```python
from build123d import *

# Parameters (mm, degrees)
F1_DEPTH = 2.25
F2_DEPTH = 2.55


with BuildPart() as f1:
    # F0 (on Top) → F1 (new body)
    with BuildSketch(Plane.XY):
        with BuildLine():
            ThreePointArc((-4.875, -1.5), (0, -0.2318236393), (4.875, -1.5))
            Line((4.875, -1.5), (4.875, 1.5))
            Line((4.875, 1.5), (-4.875, 1.5))
            Line((-4.875, 1.5), (-4.875, -1.5))
        make_face()
        with BuildLine():
            Line((1.0935325176, -1.5), (4.875, -1.5))
            ThreePointArc((4.875, -1.5), (0, -0.2318236393), (-4.875, -1.5))
            Line((-4.875, -1.5), (-1.0935325176, -1.5))
            ThreePointArc((-1.0935325176, -1.5), (0, -1.4318236393), (1.0935325176, -1.5))
        make_face()
    extrude(amount=F1_DEPTH)

    # F0 (on Top) → F2 (join)
    with BuildSketch(Plane.XY):
        with BuildLine():
            ThreePointArc((10.0040881804, -10.2359118196), (8.6270420829, -5.1707439823), (4.875, -1.5))
            Line((4.875, -1.5), (1.0935325176, -1.5))
            ThreePointArc((1.0935325176, -1.5), (6.6007395571, -4.4099178283), (8.8040881804, -10.2359118196))
            ThreePointArc((8.8040881804, -10.2359118196), (-5.8259939913, -16.8366513767), (-1.0935325176, -1.5))
            Line((-1.0935325176, -1.5), (-4.875, -1.5))
            ThreePointArc((-4.875, -1.5), (-5.0651678374, -18.8629539025), (10.0040881804, -10.2359118196))
        make_face()
    extrude(amount=F2_DEPTH)


solid = f1.part
```
The listing builds one solid part. Answer for the finished solid, in the listing's coordinates (mm). A direction names the side the tool comes from. Give positions to 0.01 mm unless a question says otherwise; leave off trailing zeros. Order: outer loops, then holes, each group sorted by start corner. A loop starts at its lowest first (then second) coordinate and runs counter-clockwise, first axis right, second up. Notation, with made-up numbers: (11, -14.5) -> (24, -14.5) arc R13 cw to (24, -6.5) -> close; hole circle Ø6 at (-27, -6). An arc over 180 degrees is marked (long way). Answer as a JSON object with one key per item and string values. Group by question number.
Item 1: The part is cut by section A-A on x = 0. Write down the section's boundary in (y, z).
Item 2: The part is cut by section C-C on z = 1.8. Write down the section's boundary in (x, y) (3 decimals), and give its area (3 significant figures).
Item 3: The part is cut by section B-B on y = -5.5. Write down the section's boundary in (x, z), and give its area (3 significant figures).
Item 4: Flat-ended cylindrical pins translate along their axes: pin 1 (1 mm diameter, centred on y = -4.5, z = 2, fed in from +X); pin 2 (2.5 mm diameter, centred on x = 1, y = 0.5, fed in from +Z); pin 3 (1.5 mm diameter, centred on y = -15, z = 1, fed in from +X); pin 4 (8 mm diameter, centred on x = 2, y = -8, fed in from -Z). Find the tip coordinate at first contact, or state that the pin passes through.
Item 5: Consider L1, parallel to Y at x = 0, z = 1.6; L2, parallel to X at y = -18.25, z = 0.2; L3, parallel to Y at x = 0.75, z = 2.2. Determine where each line is inside the solid, lowest interval first. Write a range as from..to.
Item 6: A tool of negligible diameter and unlimited length cuts with its end or side. For faces 1 (the flat face through (0, 1.5, 1)), 2 (the flat face through (0, 0, 2.25)), 3 (the flat face through (-0.8, -19.2, 2.55)), 4 (the flat face through (4.875, 0, 1)), 5 (the flat face through (-4.875, 0, 1)), from which of +Z, -Z, +X, -X, +Y, -Y can it reach the whole face along a straight path? Write none if from no direction.
Result set:
{
 "1": {"outline": "(-20.24, 0) -> (-19.04, 0) -> (-19.04, 2.55) -> (-20.24, 2.55) -> close; (-1.43, 0) -> (1.5, 0) -> (1.5, 2.25) -> (-1.43, 2.25) -> close"},
 "2": {"outline": "(-4.875, -1.5) arc R10.004 ccw (long way) to (4.875, -1.5) -> (4.875, 1.5) -> (-4.875, 1.5) -> close; hole circle Ø17.608 at (0, -10.236)", "area": "91.8 mm²"},
 "3": {"outline": "(-8.81, 0) -> (-7.42, 0) -> (-7.42, 2.55) -> (-8.81, 2.55) -> close; (7.42, 0) -> (8.81, 0) -> (8.81, 2.55) -> (7.42, 2.55) -> close", "area": "7.09 mm²"},
 "4": {"pin 1": "x = 8.52", "pin 2": "z = 2.25", "pin 3": "x = 9.16", "pin 4": "through"},
 "5": {"L1": "-20.24..-19.04, -1.43..1.5", "L2": "-5.99..-3.65, 3.65..5.99", "L3": "-20.21..-19.01, -1.46..1.5"},
 "6": {"face 1": "+Z, -Z, +X, -X, +Y", "face 2": "+Z, +X, -X, +Y", "face 3": "+Z, +X, -X, +Y, -Y", "face 4": "+Z, -Z, +X, +Y", "face 5": "+Z, -Z, -X, +Y"}
}
